CAD build for the part. Positions are in the model's coordinates, mm. Coordinates: 2 decimals unless noted, no trailing zeros. Loops run counter-clockwise (first coordinate to the right, second up) from the corner with the lowest first, then second, coordinate; pieces in that order, holes last. Notation, with made-up numbers: (12.5, -9.5) -> (53.5, -9.5) arc R26 cw to (53.5, 10.5) -> close; hole circle Ø10 at (58.5, 74). An arc over 180 degrees is marked (long way). Write each question's results on one line, items separated by ' | '.
```python
from build123d import *

# Parameters (mm, degrees)
F1_DEPTH = 2
F2_DEPTH = 1.5
F3_SIZE2 = 5
F3_SIZE  = 1.49
F4_SIZE2 = 5
F4_SIZE  = 1.49
F5_SIZE2 = 5
F5_SIZE  = 1.49
F6_SIZE  = 1.99999
F7_R     = 2.5
F8_DEPTH = 1.4


# Not quite as in the source:
# - a fillet or chamfer is up to 0.001 mm smaller than in the source, because OpenCascade refuses the exact size


with BuildPart() as f1:
    # F0 (on Top) → F1 (new body)
    with BuildSketch(Plane.XY):
        Polygon((0, 5), (0, 0), (0, -5), (7.3, -5), (7.3, -3), (16.8, -3), (16.8, -8.3876634017), (20.6713799321, -7.1317504184), (31.9639886349, -8.4706461057), (27.770944377, -5.5), (31.6675294298, 0), (27.770944377, 5.5), (31.9639886349, 8.4706461057), (20.6713799321, 7.1317504184), (16.8, 8.3876634017), (16.8, 3), (7.3, 3), (7.3, 5), align=None)
    extrude(amount=-F1_DEPTH)

    # F0 (on Top) → F2 (join)
    with BuildSketch(Plane.XY):
        Polygon((0, 5), (0, 0), (0, -5), (7.3, -5), (7.3, -3), (16.8, -3), (16.8, -8.3876634017), (20.6713799321, -7.1317504184), (31.9639886349, -8.4706461057), (27.770944377, -5.5), (31.6675294298, 0), (27.770944377, 5.5), (31.9639886349, 8.4706461057), (20.6713799321, 7.1317504184), (16.8, 8.3876634017), (16.8, 3), (7.3, 3), (7.3, 5), align=None)
        Polygon((67.1471691582, 5.5), (27.770944377, 5.5), (31.6675294298, 0), (27.770944377, -5.5), (67.4096829149, -5.5), (68.6014365075, -4.5), (100, -4.5), (116.0886735, 9), (71.3183067322, 9), align=None)
    extrude(amount=-F2_DEPTH)

    # F3
    f3_edges = [f1.edges().sort_by_distance(p)[0] for p in [
        (84.300718, -4.5, -1.5),
    ]]
    f3_side = f1.faces().sort_by_distance((84.300718, -4.5, -0.75))[0]
    chamfer(f3_edges, length=F3_SIZE, length2=F3_SIZE2, reference=f3_side)

    # F4
    f4_edges = [f1.edges().sort_by_distance(p)[0] for p in [
        (47.590314, -5.5, -1.5),
    ]]
    f4_side = f1.faces().sort_by_distance((47.590314, -5.5, -0.75))[0]
    chamfer(f4_edges, length=F4_SIZE, length2=F4_SIZE2, reference=f4_side)

    # F5
    f5_edges = [f1.edges().sort_by_distance(p)[0] for p in [
        (111.023721, 4.75, -1.5),
    ]]
    f5_side = f1.faces().sort_by_distance((109.409925, 3.395865, -0.692895))[0]
    chamfer(f5_edges, length=F5_SIZE, length2=F5_SIZE2, reference=f5_side)

    # F6 (size 2 in the source; OpenCascade refuses exactly that, so slightly less here)
    f6_edges = [f1.edges().sort_by_distance(p)[0] for p in [
        (7.3, 5, -1),
        (7.3, -5, -1),
    ]]
    chamfer(f6_edges, length=F6_SIZE)

    # F7 (on Top) → F8 (cut)
    with BuildSketch(Plane.XY):
        with Locations((22, 0)):
            Circle(F7_R)
        with Locations((90, 3.9548357017)):
            Circle(F7_R)
    extrude(amount=-F8_DEPTH, mode=Mode.SUBTRACT)


solid = f1.part
```
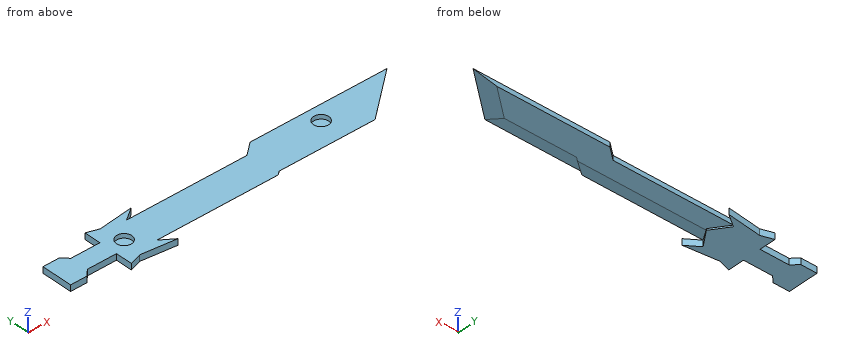
Q1. Cut at A-A on z = -1. Give the number of separate pieces and of enclosed holes in the cut face, and give its area (3 significant figures).
Results are:
separate pieces: 1 | enclosed holes: 2 | area: 952 mm^2
Q2. Drop flat-ended pins along their axis: pin 1 (1 mm diameter, centred on y = 1.5, z = -1.5, fed in from -X); pin 2 (5 mm diameter, centred on x = 56, y = 2, fed in from -Z); pin 3 (0.6 mm diameter, centred on x = 2, z = -1.5, fed in from +Y); pin 4 (1.5 mm diameter, centred on x = 89.5, y = 3.5, fed in from +Z). Give the stop position or say it passes through.
Results are:
pin 1: x = 0 | pin 2: z = -1.5 | pin 3: y = 5 | pin 4: z = -1.4
Q3. Wall check: L1, parallel to Y at x = 22, z = -0.6; L2, parallel to X at y = -3.5, z = -0.9; L3, parallel to Z at x = 81, y = 3. Give the ranges that are in metal, low to high. Write a range as from..to.
Results are:
L1: -7.29..-2.5, 2.5..7.29 | L2: 0..6.8, 16.8..29.19 | L3: -1.5..0
Q4. Cut at D-D on x = 22. Write the cut outline in (y, z).
Results are:
outline: (-7.29, -2) -> (7.29, -2) -> (7.29, 0) -> (2.5, 0) -> (2.5, -1.4) -> (-2.5, -1.4) -> (-2.5, 0) -> (-7.29, 0) -> close
